from build123d import *

# Parameters (mm, degrees)
F1_DEPTH = 10
F0_W     = 36
F0_H     = 62.5223250638
F2_DEPTH = 40
F3_R     = 5.5
F4_DEPTH = 25
F5_R     = 6
F6_DEPTH = 25


with BuildPart() as f1:
    # F0 (on Front) → F1 (new body)
    with BuildSketch(Plane.XZ):
        Polygon((20, 72.5223250638), (0, 10), (20, 10), align=None)
    extrude(amount=F1_DEPTH)



with BuildPart() as f1b:
    # F0 (on Front) → F1, piece 2 (new body)
    with BuildSketch(Plane.XZ):
        with Locations((48, 31.2611625319)):
            Rectangle(F0_W, F0_H)
    extrude(amount=F1_DEPTH)


with BuildPart() as f1c:
    # F0 (on Front) → F1, piece 3 (new body)
    with BuildSketch(Plane.XZ):
        Polygon((96, 9.5949610695), (76, 72.5223250638), (76, 9.7544647339), align=None)
    extrude(amount=F1_DEPTH)


with BuildPart() as f1_1:
    add(f1.part)

    add(f1b.part)  # F2 merges F1b

    add(f1c.part)  # F2 merges F1c
    # F0 (on Front) → F2 (join)
    with BuildSketch(Plane.XZ):
        Polygon((0, 10), (0, 0), (30, 0), (30, 62.5223250638), (66, 62.5223250638), (66, 0), (96, 0), (96, 9.5949610695), (76, 9.7544647339), (76, 72.5223250638), (20, 72.5223250638), (20, 10), align=None)
    extrude(amount=F2_DEPTH)

    # F3 (on Top) → F4 (cut)
    with BuildSketch(Plane.XY):
        with Locations((10, -28)):
            Circle(F3_R)
        with Locations((86, -28)):
            Circle(F3_R)
    extrude(amount=F4_DEPTH, mode=Mode.SUBTRACT)

    # F5 (on face) → F6 (cut)
    with BuildSketch(Plane.XY.offset(72.5223250638)):
        with Locations((48, -25)):
            Circle(F5_R)
    extrude(amount=-F6_DEPTH, mode=Mode.SUBTRACT)


solid = f1_1.part
Verification items for the finished model (mm, model axes). A direction names the side the tool comes from. Coordinates: 2 decimals unless noted, no trailing zeros. Order: outer loops, then holes, each group sorted by start corner. A loop starts at its lowest first (then second) coordinate and runs counter-clockwise, first axis right, second up. Notation, with made-up numbers: (-11, -37) -> (-1, -37) arc R30 ccw to (-1, -9) -> close; hole circle Ø8 at (85, 43). An arc over 180 degrees is marked (long way). Put each result on its own line as item: value. Start each with the question number.
1. Cross-section at B-B, the plane y = -26.5. Record the boundary of the cut face in (x, z).
2. Cross-section at C-C, the plane y = -11.5. Record the boundary of the cut face in (x, z), then the cut area to 3 significant figures.
3. Cross-section at A-A, the plane x = 48. Record the boundary of the cut face in (y, z), then the cut area to 3 significant figures.
4. Go/stop test with flat-tipped pins: pin 1 Ø16 at (x, z) = (90.5, 45.5) entering from -Y; pin 2 Ø15 at (y, z) = (-24, 34) entering from -X; pin 3 Ø15 at (y, z) = (-27, 43) entering from +X; pin 4 Ø7 at (x, y) = (48, -25) entering from -Z. Record where each tip stops, or that it passes through.
5. Cross-section at D-D, the plane z = 52.5. Record the boundary of the cut face in (x, y), then the cut area to 3 significant figures.
6. Material ranges on L1, parallel to X at y = -28, z = 5.75; L2, parallel to X at y = -16.5, z = 49; L3, parallel to Y at x = 10, z = 6, recorded low to high. Write a range as [from, to].
7. Mould release check, pull along Y, two halves, no side actions. Record for faces 4 (the flat face through (10, -21, 10)), 5 (the flat face through (14, -10, 28)), 6 (the cylindrical face through (12.957, -23.362, 4.93)), 7 (the cylindrical face through (42, -25, 68)): released by +Y, released by -Y, zero draft, split by the parting line, or undercut.
8. Access from +Z, -Z, +X, -X, +Y, -Y to the whole of each face (thin tool, end or side, straight path). Record for faces 1 (the flat face through (48, -18, 62.522)), 2 (the flat face through (48, -15, 72.522)), 3 (the flat face through (76, -25, 41)).
Computed:
1. outline: (0, 0) -> (4.71, 0) -> (4.71, 10) -> (0, 10) -> close; (15.29, 0) -> (30, 0) -> (30, 62.52) -> (42.19, 62.52) -> (42.19, 72.52) -> (20, 72.52) -> (20, 10) -> (15.29, 10) -> close; (53.81, 62.52) -> (66, 62.52) -> (66, 0) -> (80.71, 0) -> (80.71, 9.72) -> (76, 9.75) -> (76, 72.52) -> (53.81, 72.52) -> close; (91.29, 0) -> (96, 0) -> (96, 9.59) -> (91.29, 9.63) -> close
2. outline: (0, 0) -> (30, 0) -> (30, 62.52) -> (66, 62.52) -> (66, 0) -> (96, 0) -> (96, 9.59) -> (76, 9.75) -> (76, 72.52) -> (20, 72.52) -> (20, 10) -> (0, 10) -> close
2. area: 2,200 mm2
3. outline: (-40, 62.52) -> (-31, 62.52) -> (-31, 72.52) -> (-40, 72.52) -> close; (-19, 62.52) -> (-10, 62.52) -> (-10, 0) -> (0, 0) -> (0, 72.52) -> (-19, 72.52) -> close
3. area: 905 mm2
4. pin 1: y = -10
4. pin 2: x = 20
4. pin 3: x = 76
4. pin 4: through
5. outline: (13.6, -10) -> (20, -10) -> (20, -40) -> (30, -40) -> (30, -10) -> (66, -10) -> (66, -40) -> (76, -40) -> (76, -10) -> (82.36, -10) -> (82.36, 0) -> (13.6, 0) -> close
5. area: 1,290 mm2
6. L1: [0, 4.5], [15.5, 30], [66, 80.5], [91.5, 96]
6. L2: [20, 30], [66, 76]
6. L3: [-40, -33.5], [-22.5, 0]
7. face 4: zero draft
7. face 5: released by -Y
7. face 6: undercut
7. face 7: undercut
8. face 1: -Z, -Y
8. face 2: +Z, +X, -X, +Y, -Y
8. face 3: +Z, +X, -Y
